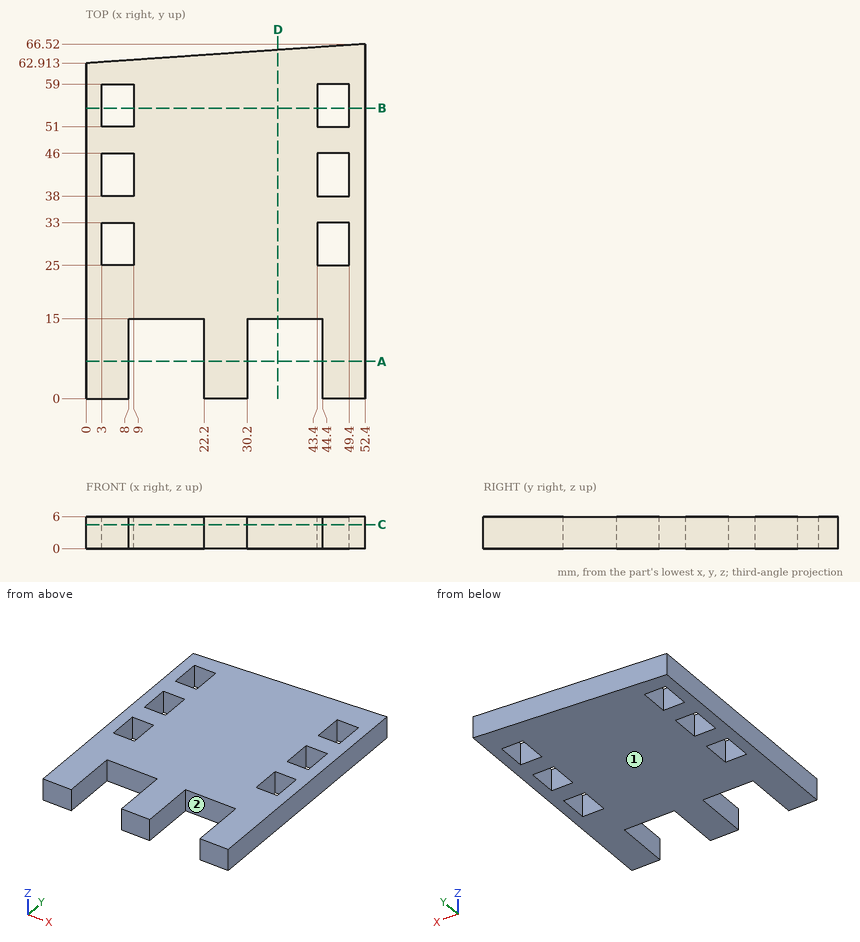
Design review of the part shown in the three views and the two pictorial views. Dimensions are in mm from the part's minimum x, y and z. A direction names the side the tool comes from. Round coordinates to 2 decimals unless told otherwise and drop trailing zeros. Write each loop counter-clockwise with the first axis right and the second up, starting at its lowest first coordinate (ties: lowest second). Pieces come first, ordered by that corner, then holes. Notation, with made-up numbers: (5.25, 18.25) - (39.25, 18.25) arc R19 ccw to (39.25, 51.25) - close; hole circle Ø8 at (13, 58). An arc over 180 degrees is marked (long way). Write item = value, one per line. Start each with the question number.
1. Consider section D-D on x = 36. State the section outline as (y, z) points.
2. Wall thickness on L1, parallel to X at y = 7, z = 1.4; L2, parallel to X at y = 42.5, z = 1.4; L3, parallel to Y at x = 19, z = 4.05: over which ranges is each line inside the solid? List them lowest first.
3. Consider section B-B on y = 54.5. State the section outline as (x, z) points.
4. Consider section C-C on z = 4.5. Give the number of separate pieces and of enclosed holes in the cut face, plus the area to 3 significant figures.
5. For pin 1 Ø2 at (x, z) = (9.5, 1) entering from -Y; pin 2 Ø3 at (x, z) = (6.5, 3) entering from +Y, all flat-tipped, find the tip position at first contact; note any pin that passes through.
6. Consider section A-A on y = 7. State the section outline as (x, z) points.
7. For the marked faces 1 and 2, list the 3-axis set-ups (+Z, -Z, +X, -X, +Y, -Y) from which the entire face can be reached by the end or side of a thin tool; tool diameter is ignored.
Evaluation:
q1.outline = (15, 0) - (65.39, 0) - (65.39, 6) - (15, 6) - close
q2.L1 = 0 to 8, 22.2 to 30.2, 44.4 to 52.4
q2.L2 = 0 to 3, 9 to 43.4, 49.4 to 52.4
q2.L3 = 15 to 64.22
q3.outline = (0, 0) - (3, 0) - (3, 6) - (0, 6) - close; (9, 0) - (43.4, 0) - (43.4, 6) - (9, 6) - close; (49.4, 0) - (52.4, 0) - (52.4, 6) - (49.4, 6) - close
q4.separate_pieces = 1
q4.enclosed_holes = 6
q4.area = 2,680 mm2
q5.pin_1 = 15
q5.pin_2 = 63.46
q6.outline = (0, 0) - (8, 0) - (8, 6) - (0, 6) - close; (22.2, 0) - (30.2, 0) - (30.2, 6) - (22.2, 6) - close; (44.4, 0) - (52.4, 0) - (52.4, 6) - (44.4, 6) - close
q7.face_1 = -Z, +X, -X, +Y, -Y
q7.face_2 = +Z, -Z, -Y
